```python
from build123d import *

# Parameters (mm, degrees)
SKETCH_1_W          = 30
SKETCH_1_H          = 10
SKETCH_1_W_2        = 27
SKETCH_1_H_2        = 7
EXTRUDE_1_DEPTH     = 250
SKETCH_2_R          = 1.6
CUT_EXTRUDE_1_DEPTH = 252.843205189
SKETCH_6_W          = 28
SKETCH_6_H          = 8
CUT_EXTRUDE_5_DEPTH = 330
SKETCH_8_W          = 4
SKETCH_8_H          = 25
CUT_EXTRUDE_6_DEPTH = 5
SKETCH_10_R         = 1.65
SKETCH_10_W         = 40
SKETCH_10_H         = 39.7
CUT_EXTRUDE_7_DEPTH = 25
FILLET_1_R          = 2
SKETCH_11_R         = 1.2
CUT_EXTRUDE_8_DEPTH = 25


with BuildPart() as part:
    # 草图1 → 凸台-拉伸1 (new body)
    with BuildSketch(Plane.XY):
        Rectangle(SKETCH_1_W, SKETCH_1_H)
        Rectangle(SKETCH_1_W_2, SKETCH_1_H_2, mode=Mode.SUBTRACT)
    extrude(amount=EXTRUDE_1_DEPTH)

    # 草图2 → 切除-拉伸1 (cut, through all)
    with BuildSketch(Plane(origin=(15, 0, 0), x_dir=(0, 0, -1), z_dir=(1, 0, 0))):
        with Locations((-240, 0)):
            Circle(SKETCH_2_R)
        with Locations((-220, 0)):
            Circle(SKETCH_2_R)
        with Locations((-200, 0)):
            Circle(SKETCH_2_R)
        with Locations((-50, 0)):
            Circle(SKETCH_2_R)
        with Locations((-30, 0)):
            Circle(SKETCH_2_R)
        with Locations((-10, 0)):
            Circle(SKETCH_2_R)
    extrude(amount=-CUT_EXTRUDE_1_DEPTH, mode=Mode.SUBTRACT)

    # 草图6 → 切除-拉伸5 (cut)
    with BuildSketch(Plane(origin=(0, 0, 0), x_dir=(-1, 0, 0), z_dir=(0, 0, -1))):
        Rectangle(SKETCH_6_W, SKETCH_6_H)
    extrude(amount=-CUT_EXTRUDE_5_DEPTH, mode=Mode.SUBTRACT)

    # 草图8 → 切除-拉伸6 (cut)
    with BuildSketch(Plane(origin=(0, 5, 0), x_dir=(1, 0, 0), z_dir=(0, 1, 0))):
        with BuildLine():
            Line((-10, -150), (-10, -155))
            ThreePointArc((-10, -155), (-7.071067812, -162.071067812), (0, -165))
            Line((0, -165), (0, -85))
            ThreePointArc((0, -85), (-7.071067812, -87.928932188), (-10, -95))
            Line((-10, -95), (-10, -100))
            Line((-10, -100), (-10, -125))
            Line((-10, -125), (-10, -150))
        make_face()
        with BuildLine():
            Line((0, -85), (0, -165))
            ThreePointArc((0, -165), (7.071067812, -162.071067812), (10, -155))
            Line((10, -155), (10, -150))
            Line((10, -150), (10, -125))
            Line((10, -125), (10, -100))
            Line((10, -100), (10, -95))
            ThreePointArc((10, -95), (7.071067812, -87.928932188), (0, -85))
        make_face()
        with Locations((12, -112.5)):
            Rectangle(SKETCH_8_W, SKETCH_8_H)
        with Locations((12, -137.5)):
            Rectangle(SKETCH_8_W, SKETCH_8_H)
        with Locations((-12, -112.5)):
            Rectangle(SKETCH_8_W, SKETCH_8_H)
        with Locations((-12, -137.5)):
            Rectangle(SKETCH_8_W, SKETCH_8_H)
    extrude(amount=-CUT_EXTRUDE_6_DEPTH, mode=Mode.SUBTRACT)

    # 草图10 → 切除-拉伸7 (cut)
    # profile 1 of 4: a face of its own
    with BuildSketch(Plane.XZ.offset(5)):
        with Locations(Location((-12, 115, 0), (0, 0, 270))):
            Circle(SKETCH_10_R)
    # profile 2 of 4: a face of its own
    with BuildSketch(Plane.XZ.offset(5)):
        with Locations(Location((-12, 135, 0), (0, 0, 270))):
            Circle(SKETCH_10_R)
    # profile 3 of 4: a face of its own
    with BuildSketch(Plane.XZ.offset(5)):
        with Locations(Location((11.7, 125, 0), (0, 0, 270))):
            Circle(SKETCH_10_R)
    # profile 4 of 4: a face of its own
    with BuildSketch(Plane.XZ.offset(5)):
        with Locations((-84.485896168, 54.669789624)):
            Rectangle(SKETCH_10_W, SKETCH_10_H)
        with Locations((-84.485896168, 42.819789624)):
            Circle(SKETCH_10_R, mode=Mode.SUBTRACT)
        with Locations((-94.485896168, 66.519789624)):
            Circle(SKETCH_10_R, mode=Mode.SUBTRACT)
        with Locations((-74.485896168, 66.519789624)):
            Circle(SKETCH_10_R, mode=Mode.SUBTRACT)
    extrude(amount=-CUT_EXTRUDE_7_DEPTH, mode=Mode.SUBTRACT)

    # 圆角1
    fillet_1_edges = [part.edges().sort_by_distance(p)[0] for p in [
        (-14, 4.5, 150),
        (14, 4.5, 150),
        (14, 4.5, 100),
        (-14, 4.5, 100),
    ]]
    fillet(fillet_1_edges, radius=FILLET_1_R)
    fillet_1_2_edges = [part.edges().sort_by_distance(p)[0] for p in [
        (10, 4.5, 100),
        (-10, 4.5, 100),
        (-10, 4.5, 150),
        (10, 4.5, 150),
    ]]
    fillet(fillet_1_2_edges, radius=FILLET_1_R - 0.0001)  # a hair under: the kernel refuses the full size

    # 草图11 → 切除-拉伸8 (cut)
    with BuildSketch(Plane.XZ.offset(5)):
        with Locations(Location((-10, 142.5, 0), (0, 0, 270))):
            Circle(SKETCH_11_R)
        with Locations(Location((10, 142.5, 0), (0, 0, 270))):
            Circle(SKETCH_11_R)
        with Locations(Location((10, 107.5, 0), (0, 0, 270))):
            Circle(SKETCH_11_R)
        with Locations(Location((-10, 107.5, 0), (0, 0, 270))):
            Circle(SKETCH_11_R)
    extrude(amount=-CUT_EXTRUDE_8_DEPTH, mode=Mode.SUBTRACT)


solid = part.part
```
Design review of the part built by this model. Coordinates are the model's own, in mm. A direction names the side the tool comes from. Coordinates: 2 decimals unless noted, no trailing zeros. Write each loop counter-clockwise with the first axis right and the second up, starting at its lowest first coordinate (ties: lowest second). Pieces come first, ordered by that corner, then holes.
1) Mouldability with a two-part tool opening along Y and no side actions: class faces 1 (the flat face through (15, 0, 123)), 2 (the flat face through (-14, 0, 123)), 3 (the flat face through (0, 4, 50)), 4 (the flat face through (-10.2, 5, 95.5)) as +Y half, -Y half, draft (parallel to the pull), parting line (faces both ways), or undercut.
2) To check wall thickness, follow L1, parallel to X at y = 2.75, z = 130.5; L2, parallel to X at y = -4.6, z = 115; L3, parallel to Y at x = 6.5, z = 12. State the ranges of each line that lie inside material, in increasing order.
3) Add section C-C (z = 92.5). Write out the cut boundary in (x, y).
4) Add section B-B (z = 39). Write out the cut boundary in (x, y), plus the area to 3 significant figures.
5) Machinability: for faces 5 (the flat face through (0, 4, 210)), 6 (the flat face through (-0.1, -4.4, 0)), which of the approach directions +Z, -Z, +X, -X, +Y, -Y give a long, thin tool a straight path to every point of the face, cutting with its end or side? Answer none if there is none.
6) Insertion check: pin 1 (4 mm diameter, centred on x = -10, z = 107.5, fed in from +Y). The pin has a flat end and moves straight along its axis. Give the tip position at first contact, or say it passes through.
7) Add section A-A (x = -3.25). Write out the cut boundary in (y, z).
Check result:
1. face 1: draft
1. face 2: undercut
1. face 3: undercut
1. face 4: +Y half
2. L1: x = -15 to -14, 14 to 15
2. L2: x = -15 to -13.65, -10.35 to 15
2. L3: y = -5 to -4, 4 to 5
3. outline: (-15, -5) - (15, -5) - (15, 5) - (9.68, 5) - (9.68, 4) - (14, 4) - (14, -4) - (-14, -4) - (-14, 4) - (-9.68, 4) - (-9.68, 5) - (-15, 5) - close
4. outline: (-15, -5) - (15, -5) - (15, 5) - (-15, 5) - close; hole (-14, -4) - (14, -4) - (14, 4) - (-14, 4) - close
4. area: 76.0 mm2
5. face 5: +Z, -Z
5. face 6: -Z, +X, -X, +Y, -Y
6. pin 1: stops at y = -4
7. outline: (-5, 0) - (-4, 0) - (-4, 250) - (-5, 250) - close; (4, 0) - (5, 0) - (5, 85.54) - (4, 85.54) - close; (4, 164.46) - (5, 164.46) - (5, 250) - (4, 250) - close
